Source: CAD feature listing. Evaluate the final solid. Frame: model axes, mm. A direction names the side the tool comes from. Round coordinates to 2 decimals unless told otherwise and drop trailing zeros. One line per item, written item: value.
from build123d import *

# Parameters (mm, degrees)
F1_DEPTH  = 20
F3_DEPTH  = 21
F4_T      = -2.5
F6_W      = 10
F6_H      = 5.5
F7_DEPTH  = 25
F8_W      = 55.2565678954
F8_H      = 1.5035793185
F9_DEPTH  = 2
F10_R     = 2
F12_DEPTH = 70
F14_DEPTH = 25
F16_DEPTH = 25
F17_W     = 13.128624599
F17_H     = 37
F18_DEPTH = 13.5
F19_W     = 13.128624711
F19_H     = 37
F20_DEPTH = 13.5
F21_W     = 57.774464488
F21_H     = 1
F21_W_2   = 57.7263757586
F21_H_2   = 1.2739617378
F22_DEPTH = 13.5


with BuildPart() as f1:
    # F0 (on Front) → F1 (new body, symmetric)
    with BuildSketch(Plane.XZ):
        with BuildLine():
            Line((31.387232244, -27.2523891181), (31.387232244, 27.0644389093))
            ThreePointArc((31.387232244, 27.0644389093), (0, 58.4516711533), (-31.387232244, 27.0644389093))
            Line((-31.387232244, 27.0644389093), (-31.387232244, -27.2523891181))
            Line((-31.387232244, -27.2523891181), (31.387232244, -27.2523891181))
        make_face()
    extrude(amount=F1_DEPTH, both=True)

    # F2 (on Front) → F3 (join, symmetric)
    with BuildSketch(Plane.XZ):
        Polygon((31.1992858725, -26.8764924258), (-31.1992857605, -26.8764924258), (-44.5384809197, -26.8764924258), (-44.3942922286, -42.8813642573), (5.62e-08, -43.0360519628), (44.3942923407, -42.8813642573), (44.5384810317, -26.8764924258), align=None)
    extrude(amount=F3_DEPTH, both=True)

    # F4
    f4_openings = [f1.faces().sort_by_distance(p)[0] for p in [
        (-22.197146, 0, -42.958708),
        (22.197146, 0, -42.958708),
    ]]
    offset(amount=F4_T, openings=f4_openings, kind=Kind.INTERSECTION)

    # F6 (on face) → F7 (cut)
    with BuildSketch(Plane.XZ.offset(20)):
        Polygon((2.3308762088, 51.4463313338), (-3.1691237912, 51.4463313338), (-3.1691237912, 43.8206121624), (-3.1691237912, 38.3206121624), (-3.1691237912, 13.312992971), (2.3308762088, 13.312992971), (2.3308762088, 38.3206121624), (2.3308762088, 43.8206121624), align=None)
        with Locations((-8.1691237912, 41.0706121624)):
            Rectangle(F6_W, F6_H)
        with Locations((7.3308762088, 41.0706121624)):
            Rectangle(F6_W, F6_H)
    extrude(amount=-F7_DEPTH, mode=Mode.SUBTRACT)

    # F8 (on face) → F9 (join)
    with BuildSketch(Plane.XZ.offset(20)):
        with Locations((0, 11.088903062)):
            Rectangle(F8_W, F8_H)
    extrude(amount=F9_DEPTH)

    # F10
    f10_edges = [f1.edges().sort_by_distance(p)[0] for p in [
        (0, -20, 58.451671),
        (0, 20, 58.451671),
    ]]
    fillet(f10_edges, radius=F10_R)

    # F11 (on face) → F12 (cut)
    with BuildSketch(Plane.YZ.offset(31.387232244)):
        Polygon((-4.1348445229, -5.0745825283), (-13.156324625, -10.9009547159), (-2.2320076807, -6.3103797534), (-6.5781623125, 7.1420050226), (-4.698687233, 20.8621732891), (-8.081741631, 7.1420050226), align=None)
    extrude(amount=-F12_DEPTH, mode=Mode.SUBTRACT)

    # F13 (on face) → F14 (cut)
    with BuildSketch(Plane.XZ.offset(20)):
        Polygon((-11.2768495455, -18.6068024486), (-16.1634851247, -26.6885459423), (-8.6455848068, -16.915274784), (-13.156324625, -15.2237480506), (0, -11.4647978917), (-18.4239908566, -14.2852751634), align=None)
    extrude(amount=-F14_DEPTH, mode=Mode.SUBTRACT)

    # F15 (on face) → F16 (cut)
    with BuildSketch(Plane.XZ.offset(20)):
        Polygon((20.1853319103, 40.9697728612), (22.5537028164, 45.6712394953), (17.1032212675, 41.1605015397), (21.5089086938, 35.8369561988), (16.9085077893, 32.0297324177), (24.4331751019, 35.8369561988), align=None)
    extrude(amount=-F16_DEPTH, mode=Mode.SUBTRACT)

    # F17 (on face) → F18 (join)
    with BuildSketch(Plane(origin=(0, 0, -29.3764924258), x_dir=(1, 0, 0), z_dir=(0, 0, -1))):
        with Locations((-35.4515445435, 0)):
            Rectangle(F17_W, F17_H)
    extrude(amount=F18_DEPTH)

    # F19 (on face) → F20 (join)
    with BuildSketch(Plane(origin=(0, 0, -29.3764924258), x_dir=(1, 0, 0), z_dir=(0, 0, -1))):
        with Locations((35.4515445995, 0)):
            Rectangle(F19_W, F19_H)
    extrude(amount=F20_DEPTH)

    # F21 (on face) → F22 (join)
    with BuildSketch(Plane(origin=(0, 0, -29.3764924258), x_dir=(1, 0, 0), z_dir=(0, 0, -1))):
        with Locations((0, 18)):
            Rectangle(F21_W, F21_H)
        with Locations((0.0108480453, -17.9641498253)):
            Rectangle(F21_W_2, F21_H_2)
    extrude(amount=F22_DEPTH)


solid = f1.part
1. Pull-direction query (X, two-part tool) for faces 1 (the face through (-8, -19, 43.821)), 2 (the face through (-1, 21, -35)), 3 (the face through (-12.457, -18.768, -21.87)), 4 (the face through (0.69, -0.252, 58.444)); classes: released by +X, released by -X, zero draft, split by the parting line, or undercut.
Report:
face 1: undercut
face 2: zero draft
face 3: undercut
face 4: split by the parting line
2. Reachability of faces 5 (the face through (-30.12, -6.136, 1.119)), 6 (the face through (12.331, -19, 41)) from +Z, -Z, +X, -X, +Y, -Y: full face, straight path, thin tool, end or side. Return the list, or none.
Report:
face 5: +X, -X
face 6: -Y
3. Ray query, line 1 (X direction, y = -2, z = 3.5); line 2 (Y direction, x = -8, z = -24); line 3 (Z direction, x = -1.5, y = -19). Return the intervals inside material, ascending. Write a range as [from, to].
Report:
line 1: x = [-31.39, -28.89], [28.89, 31.39]
line 2: y = [-20, -17.5], [17.5, 20]
line 3: z = [-43.03, -11.89], [-11.69, 13.31], [51.45, 58.15]
4. Pin query (flat end, axial travel): pin 1 (11 mm diameter, centred on y = 3.5, z = -4.5, fed in from -X); pin 2 (12 mm diameter, centred on x = 31, y = -12, fed in from -Z); pin 3 (12 mm diameter, centred on x = 6, z = -9.5, fed in from -Y). Return the tip coordinate at first contact, or that it passes through.
Report:
pin 1: stops at x = -31.39
pin 2: stops at z = -42.88
pin 3: stops at y = -20
5. Section query D-D (x = -7). Count the separate pieces of the cut face and the enclosed holes in it, and give its area (3 significant figures).
Report:
separate pieces: 3
enclosed holes: 0
area: 613 mm2
